from build123d import *

# Parameters (mm, degrees)
SKETCH1_R               = 7.5
BOSS_EXTRUDE1_DEPTH     = 8
SKETCH2_R               = 4
CUT_EXTRUDE1_DEPTH      = 5
SKETCH3_R               = 2.5
CUT_EXTRUDE2_DEPTH      = 12
CUT_EXTRUDE3_DEPTH      = 14.285330256
CUT_EXTRUDE3_DEPTH_BACK = 14.285330256
SKETCH4_R               = 1.5


with BuildPart() as part:
    # Sketch1 → Boss-Extrude1 (new, symmetric)
    with BuildSketch(Plane(origin=(0, 0, 0), x_dir=(1, 0, 0), z_dir=(0, 1, 0))):
        with Locations(Location((0, 0, 0), (0, 0, 270))):
            Circle(SKETCH1_R)
    extrude(amount=BOSS_EXTRUDE1_DEPTH, both=True)

    # Sketch2 → Cut-Extrude1 (cut)
    with BuildSketch(Plane(origin=(0, 8, 0), x_dir=(1, 0, 0), z_dir=(0, 1, 0))):
        with Locations(Location((0, 0, 0), (0, 0, 270))):
            Circle(SKETCH2_R)
    extrude(amount=-CUT_EXTRUDE1_DEPTH, mode=Mode.SUBTRACT)

    # Sketch3 → Cut-Extrude2 (cut)
    with BuildSketch(Plane.XZ.offset(8)):
        with Locations(Location((0, 0, 0), (0, 0, 270))):
            Circle(SKETCH3_R)
    extrude(amount=-CUT_EXTRUDE2_DEPTH, mode=Mode.SUBTRACT)

    # Sketch4 → Cut-Extrude3 (cut, two sides: drawn at the far end of the back side and taken through both)
    with BuildSketch(Plane.XY.offset(-CUT_EXTRUDE3_DEPTH_BACK)):
        with Locations((0, -4)):
            Circle(SKETCH4_R)
        with Locations((0, 5)):
            Circle(SKETCH4_R)
    extrude(amount=CUT_EXTRUDE3_DEPTH + CUT_EXTRUDE3_DEPTH_BACK, mode=Mode.SUBTRACT)


solid = part.part
Work out the finished part from the listing and answer in its coordinate system (mm). A direction names the side the tool comes from. Give positions to 0.01 mm unless a question says otherwise; leave off trailing zeros. Loops run counter-clockwise (first coordinate to the right, second up) from the corner with the lowest first, then second, coordinate; pieces in that order, holes last. Notation, with made-up numbers: (44, 13) - (95, 13) arc R23 ccw to (95, 40) - close; hole circle Ø7 at (-15.75, 25). An arc over 180 degrees is marked (long way). Answer in a Markdown table with one row per item. Add a question column.
Q1. The part is cut by section A-A (z = 0). Determine the outline of the cut face in (x, y), and give its area (3 significant figures).
Q2. A tool of negligible diameter and unlimited length cuts with its end or side. For faces 1 (the flat face through (-3, 8, 3)), 2 (the cylindrical face through (-3.549, 5.535, 1.846)), from which of +Z, -Z, +X, -X, +Y, -Y can it reach the whole face along a straight path? Write none if from no direction.
Q3. Each of these flat-tipped pins is pushed along its axis until it touches: P1, Ø1, axis at x = 1.5, z = -2.5, coming from the +Y side; P2, Ø8, axis at y = -1.5, z = 4.5, coming from the -X side; P3, Ø6, axis at x = 4.5, y = 6, coming from the +Z side. Where does it stop, or does it pass through?
Q4. Determine the mould class of faces 3 (the flat face through (2, 3, 2)), 4 (the cylindrical face through (-2.87, 0.11, 6.93)), 5 (the cylindrical face through (-1.5, -3.93, -4.79)) for opening direction Z: released by +Z, released by -Z, zero draft, split by the parting line, or undercut.
Q5. The part is cut by section B-B (x = -1). Determine the outline of the cut face in (y, z), and give its area (3 significant figures).
Q6. The part is cut by section D-D (y = -0.25). Determine the outline of the cut face in (x, z).
Q7. Consider line 1 along Y through (x, z) = (0, 4.75); line 2 along X through (y, z) = (0.25, 0); line 3 along Y through (x, z) = (1, -6.25). Determine where each line is inside the solid, lowest interval first.
Q8. The part is cut by section C-C (y = 5). Determine the outline of the cut face in (x, z), and give its area (3 significant figures).
Solution:
| question | item | result |
|---|---|---|
| 1 | outline | (-7.5, -8) - (-2.5, -8) - (-2.5, 3) - (-4, 3) - (-4, 8) - (-7.5, 8) - close; (2.5, -8) - (7.5, -8) - (7.5, 8) - (4, 8) - (4, 3) - (2.5, 3) - close |
| 1 | area | 145 mm² |
| 2 | face 1 | +Z, -Z, +X, -X, +Y |
| 2 | face 2 | +Y |
| 3 | P1 | stops at y = 3 |
| 3 | P2 | stops at x = -7.48 |
| 3 | P3 | stops at z = 7.35 |
| 4 | face 3 | undercut |
| 4 | face 4 | split by the parting line |
| 4 | face 5 | zero draft |
| 5 | outline | (-8, -7.43) - (-5.12, -7.43) - (-5.12, -2.29) - (-8, -2.29) - close; (-8, 2.29) - (-5.12, 2.29) - (-5.12, 7.43) - (-8, 7.43) - close; (-2.88, -7.43) - (3.88, -7.43) - (3.88, -3.87) - (3, -3.87) - (3, -2.29) - (-2.88, -2.29) - close; (-2.88, 2.29) - (3, 2.29) - (3, 3.87) - (3.88, 3.87) - (3.88, 7.43) - (-2.88, 7.43) - close; (6.12, -7.43) - (8, -7.43) - (8, -3.87) - (6.12, -3.87) - close; (6.12, 3.87) - (8, 3.87) - (8, 7.43) - (6.12, 7.43) - close |
| 5 | area | 110 mm² |
| 6 | outline | circle Ø15 at (0, 0); hole circle Ø5 at (0, 0) |
| 7 | line 1 | y = -8 to -5.5, -2.5 to 3.5, 6.5 to 8 |
| 7 | line 2 | x = -7.5 to -2.5, 2.5 to 7.5 |
| 7 | line 3 | y = -8 to -5.12, -2.88 to 3.88, 6.12 to 8 |
| 8 | outline | (-1.5, -7.35) - (-1.5, -3.71) arc R4 cw to (-1.5, 3.71) - (-1.5, 7.35) arc R7.5 ccw to start; (1.5, -7.35) arc R7.5 ccw to (1.5, 7.35) - (1.5, 3.71) arc R4 cw to (1.5, -3.71) - close |
| 8 | area | 105 mm² |
